```python
from build123d import *

# Parameters (mm, degrees)
BOSS_EXTRUDE1_DEPTH = 8
SKETCH2_R           = 1.15
CUT_EXTRUDE1_DEPTH  = 9
SKETCH3_R           = 2
CUT_EXTRUDE2_DEPTH  = 2
SKETCH5_W           = 24
SKETCH5_H           = 44.3
SKETCH5_R           = 1.5
BOSS_EXTRUDE2_DEPTH = 5
CUT_EXTRUDE3_DEPTH  = 20
SKETCH7_W           = 8
SKETCH7_H           = 13.2
SKETCH7_R           = 1.65
SKETCH7_W_2         = 16.1
BOSS_EXTRUDE3_DEPTH = 15.55
SKETCH8_W           = 8.1
SKETCH8_H           = 5.55
CUT_EXTRUDE4_DEPTH  = 25
BOSS_EXTRUDE4_DEPTH = 10


with BuildPart() as part:
    # Sketch1 → Boss-Extrude1 (new body)
    with BuildSketch(Plane.XY):
        Polygon((0, 0), (5.866666667, 0), (5.866666667, 3), (9.066666667, 3), (9.066666667, 0), (14.933333333, 0), (14.933333333, 3), (18.133333333, 3), (18.133333333, 0), (24, 0), (24, 8), (0, 8), align=None)
    extrude(amount=-BOSS_EXTRUDE1_DEPTH)

    # Sketch2 → Cut-Extrude1 (cut, through all)
    with BuildSketch(Plane(origin=(0, 8, 0), x_dir=(1, 0, 0), z_dir=(0, 1, 0))):
        with Locations((3, 4)):
            Circle(SKETCH2_R)
        with Locations((12, 4)):
            Circle(SKETCH2_R)
        with Locations((21, 4)):
            Circle(SKETCH2_R)
    extrude(amount=-CUT_EXTRUDE1_DEPTH, mode=Mode.SUBTRACT)

    # Sketch3 → Cut-Extrude2 (cut)
    with BuildSketch(Plane(origin=(0, 8, 0), x_dir=(1, 0, 0), z_dir=(0, 1, 0))):
        with Locations((3, 4)):
            Circle(SKETCH3_R)
        with Locations((12, 4)):
            Circle(SKETCH3_R)
        with Locations((21, 4)):
            Circle(SKETCH3_R)
    extrude(amount=-CUT_EXTRUDE2_DEPTH, mode=Mode.SUBTRACT)

    # Sketch5 → Boss-Extrude2 (add)
    with BuildSketch(Plane(origin=(0, 8, 0), x_dir=(1, 0, 0), z_dir=(0, 1, 0))):
        with Locations((12, -22.15)):
            Rectangle(SKETCH5_W, SKETCH5_H)
        with Locations((9.5, -39.149393889)):
            Circle(SKETCH5_R, mode=Mode.SUBTRACT)
    extrude(amount=-BOSS_EXTRUDE2_DEPTH)

    # Sketch6 → Cut-Extrude3 (cut)
    with BuildSketch(Plane(origin=(0, 8, 0), x_dir=(1, 0, 0), z_dir=(0, 1, 0))):
        with BuildLine():
            Line((10.75, -7.8), (10.75, -21.2))
            ThreePointArc((10.75, -21.2), (8, -23.95), (5.25, -21.2))
            Line((5.25, -21.2), (5.25, -7.8))
            ThreePointArc((5.25, -7.8), (8, -5.05), (10.75, -7.8))
        make_face()
        with BuildLine():
            Line((18.75, -7.8), (18.75, -21.2))
            ThreePointArc((18.75, -21.2), (16, -23.95), (13.25, -21.2))
            Line((13.25, -21.2), (13.25, -7.8))
            ThreePointArc((13.25, -7.8), (16, -5.05), (18.75, -7.8))
        make_face()
    extrude(amount=-CUT_EXTRUDE3_DEPTH, mode=Mode.SUBTRACT)

    # Sketch7 → Boss-Extrude3 (add)
    with BuildSketch(Plane(origin=(0, 8, 0), x_dir=(1, 0, 0), z_dir=(0, 1, 0))):
        with Locations((-4, -36.02)):
            Rectangle(SKETCH7_W, SKETCH7_H)
        with Locations((-4, -33.02)):
            Circle(SKETCH7_R, mode=Mode.SUBTRACT)
        with Locations((-4, -39.02)):
            Circle(SKETCH7_R, mode=Mode.SUBTRACT)
        with Locations((32.05, -36.02)):
            Rectangle(SKETCH7_W_2, SKETCH7_H)
        with Locations((36.1, -33.02)):
            Circle(SKETCH7_R, mode=Mode.SUBTRACT)
        with Locations((36.1, -39.02)):
            Circle(SKETCH7_R, mode=Mode.SUBTRACT)
    extrude(amount=-BOSS_EXTRUDE3_DEPTH)

    # Sketch8 → Cut-Extrude4 (cut)
    with BuildSketch(Plane.XY.offset(42.62)):
        with Locations((28.05, -4.775)):
            Rectangle(SKETCH8_W, SKETCH8_H)
    extrude(amount=-CUT_EXTRUDE4_DEPTH, mode=Mode.SUBTRACT)

    # Sketch10 → Boss-Extrude4 (add)
    with BuildSketch(Plane(origin=(0, 8, 0), x_dir=(1, 0, 0), z_dir=(0, 1, 0))):
        Polygon((40.1, -29.42), (24, 8), (24, -29.42), align=None)
    extrude(amount=-BOSS_EXTRUDE4_DEPTH)


solid = part.part
```
Design review of the part built by this model. Coordinates are the model's own, in mm. A direction names the side the tool comes from. Coordinates: 2 decimals unless noted, no trailing zeros. Order: outer loops, then holes, each group sorted by start corner. A loop starts at its lowest first (then second) coordinate and runs counter-clockwise, first axis right, second up. Notation, with made-up numbers: (29.25, 78) - (64.25, 78) arc R12 cw to (64.25, 93) - close; hole circle Ø6 at (36.5, -0.5). An arc over 180 degrees is marked (long way). Answer in a Markdown table with one row per item.
(1) Clearance check with flat-ended pins moving along their axes: pin 1 (1.5 mm diameter, centred on x = 11.5, y = 2, fed in from +Z); pin 2 (1.5 mm diameter, centred on y = 5, z = 16, fed in from +X); pin 3 (13 mm diameter, centred on x = 34.5, z = 13.5, fed in from -Y). State where each tip first meets the part, or that it passes through.
Checked values:
| item | result |
|---|---|
| pin 1 | z = 0 |
| pin 2 | x = 34.65 |
| pin 3 | y = -2 |
(2) Consider section A-A on y = 1.75. Give the number of separate pieces and of enclosed holes in the cut face, plus the area to 3 significant figures.
Checked values:
| item | result |
|---|---|
| separate pieces | 4 |
| enclosed holes | 7 |
| area | 713 mm^2 |
(3) Wall thickness on line 1 along Z through (x, y) = (-4, 0.25); line 2 along X through (y, z) = (1.75, 34); line 3 along Z through (x, y) = (36.1, 3): over which ranges is each line inside the solid? List them lowest first. Write a range as from..to.
Checked values:
| item | result |
|---|---|
| line 1 | 29.42..31.37, 34.67..37.37, 40.67..42.62 |
| line 2 | -8..-5.33, -2.67..0, 24..34.77, 37.43..40.1 |
| line 3 | 20.12..31.37, 34.67..37.37, 40.67..42.62 |
(4) For faces 4 (the flat face through (32.1, -5, 36)), 5 (the flat face through (4, 6, -3)), 6 (the flat face through (12, 2, 0)), 7 (the flat face through (0, 6, 43)), 8 (the cylindrical face through (16.06, 5.54, 23.95)), list the 3-axis set-ups (+Z, -Z, +X, -X, +Y, -Y) from which the entire face can be reached by the end or side of a thin tool; tool diameter is ignored.
Checked values:
| item | result |
|---|---|
| face 4 | +Z, -Z, -Y |
| face 5 | +Y |
| face 6 | +Z, -X, -Y |
| face 7 | +Z, -X, +Y, -Y |
| face 8 | +Y, -Y |
(5) Consider section D-D on x = -4. State the section outline as (y, z) points.
Checked values:
| item | result |
|---|---|
| outline | (-7.55, 29.42) - (8, 29.42) - (8, 31.37) - (-7.55, 31.37) - close; (-7.55, 34.67) - (8, 34.67) - (8, 37.37) - (-7.55, 37.37) - close; (-7.55, 40.67) - (8, 40.67) - (8, 42.62) - (-7.55, 42.62) - close |
(6) The part is to be moulded in two halves that separate along Z. For faces 1 (the flat face through (5.867, 1, -4)), 2 (the flat face through (12, 6, 44.3)), 3 (the flat face through (18.75, 6, 14)), say which applies: released by +Z, released by -Z, zero draft, split by the parting line, or undercut.
Checked values:
| item | result |
|---|---|
| face 1 | zero draft |
| face 2 | released by +Z |
| face 3 | undercut |
(7) Consider section C-C on x = 21. State the section outline as (y, z) points, plus the area to 3 significant figures.
Checked values:
| item | result |
|---|---|
| outline | (0, -8) - (8, -8) - (8, -6) - (6, -6) - (6, -5.15) - (0, -5.15) - close; (0, -2.85) - (6, -2.85) - (6, -2) - (8, -2) - (8, 44.3) - (3, 44.3) - (3, 0) - (0, 0) - close |
| area | 264 mm^2 |
(8) Consider section B-B on y = -5. State the section outline as (x, z) points.
Checked values:
| item | result |
|---|---|
| outline | (-8, 29.42) - (0, 29.42) - (0, 42.62) - (-8, 42.62) - close; (32.1, 29.42) - (40.1, 29.42) - (40.1, 42.62) - (32.1, 42.62) - close; hole circle Ø3.3 at (-4, 33.02); hole circle Ø3.3 at (-4, 39.02); hole circle Ø3.3 at (36.1, 33.02); hole circle Ø3.3 at (36.1, 39.02) |
